Can you work these out from the model? Positions are in its coordinate system, mm. A direction names the side the tool comes from. Coordinates: 2 decimals unless noted, no trailing zeros. Order: outer loops, then holes, each group sorted by start corner. A loop starts at its lowest first (then second) coordinate and runs counter-clockwise, first axis right, second up. Notation, with made-up numbers: (-26, -19) -> (14, -19) arc R7 ccw to (14, -13) -> close; hole circle Ø1 at (85, 48). An arc over 180 degrees is marked (long way). Use a Markdown table: item, result. Add a question column.
1. If I drill on line 1 along Y through (x, z) = (-2.5, -4.25) (3 decimals); line 2 along X through (y, z) = (-20.5, -6); line 3 along Y through (x, z) = (-0.5, -4.25) (3 decimals), over which ranges is the centre line in solid material (lowest first)? Write a range as from..to.
2. For faces 1 (the cylindrical face through (-1.53, -22.37, -4.07)), 2 (the flat face through (-3, -14, -0.508)), 3 (the flat face through (-0.182, -21, -4)), 4 (the flat face through (-2, -25.175, -4)), 5 (the flat face through (-3.071, -19.626, 0.613)), which set-ups out of +Z, -Z, +X, -X, +Y, -Y let a thin tool reach every point of the face, with its end or its side?
3. For pin 1 Ø3 at (x, z) = (-2.5, -6) entering from -Y (3 decimals); pin 2 Ø3.5 at (x, y) = (-1.5, -6) entering from -Z; pin 3 Ø1.5 at (x, z) = (-1, -2.5) entering from +Y (3 decimals); pin 4 Ø3 at (x, y) = (-2, -20.5) entering from +Z, each with a flat end and sliding along its axis, tell me the tip position at first contact or that it passes through.
4. Suppose I cut it at C-C, the plane y = -21.35. List the corners of the cut face in (x, z) for me.
5. Suppose I cut it at B-B, the plane z = -3. List the corners of the cut face in (x, y) for me (3 decimals), then the cut area to 3 significant figures.
6. Suppose I cut it at A-A, the plane y = -10.75. List the corners of the cut face in (x, z) for me, then the cut area to 4 significant figures.
7. We'd pull the mould along X, two halves only. Please class faces 6 (the flat face through (-0.057, -21, 1)), 7 (the flat face through (-3.932, -21, -4)), 8 (the flat face through (-2, -25.85, 0)): pulls with the +X half, pulls with the -X half, needs draft (parallel to the pull), parting line crosses it, or undercut.
Autodesk Inventor part; units mm, degrees
ref_plane "YZ Plane" through (0, 0, 0) normal (1, 0, 0) x (0, 1, 0)
ref_plane "XZ Plane" through (0, 0, 0) normal (0, 1, 0) x (-1, 0, 0)
ref_plane "XY Plane" through (0, 0, 0) normal (0, 0, 1) x (1, 0, 0)
ref_plane "Work Plane3" through (0, -0.0002, 0) normal (0, 0, 1) x (1, 0, 0)
sketch "Sketch8" plane through (0, -0.0002, 0) normal (0, 0, 1) x (1, 0, 0)
  line L0 (-0.007, 0.0002) -> (-0.007, -15.3498)
  line L1 (-0.007, 0.0002) -> (-4.107, 0.0002)
  line L2 (-4.107, 0.0002) -> (-4.107, -11.3498)
  line L3 (-5.107, -11.3498) -> (0.993, -11.3498)
  line L4 (0.993, -11.3498) -> (0.993, 0.0002)
  line L5 (0.993, 0.0002) -> (-5.107, 0.0002)
  line L6 (-5.107, 0.0002) -> (-5.107, -11.3498)
  line L7 (-4.107, -11.3498) -> (-1.0868, -11.3498)
  point P0 (-4.107, 0.0002)
  point P1 (-0.007, 0.0002)
  point P2 (-0.007, -11.3498)
  dimension "d71" = 1
  dimension "d72" = 1
extrude "side" add sketch "Sketch8" along normal blind 1.5
sketch "Sketch14" plane through (0, -0.0002, 0) normal (0, 0, -1) x (-1, 0, 0)
  line L0 (-0.993, 0) -> (5.107, 0)
  line L1 (5.107, -11.3498) -> (-0.993, -11.3498)
  line L2 (5.107, 0.0002) -> (4.307, 0.0002)
  line L3 (4.307, 0.0002) -> (4.307, -11.3498)
  line L4 (4.307, -11.3498) -> (5.107, -11.3498)
  line L5 (5.107, -11.3498) -> (5.107, 0.0002)
  line L6 (-0.993, -11.3498) -> (-0.193, -11.3498)
  line L7 (-0.193, -11.3498) -> (-0.193, 0.0002)
  line L8 (-0.193, 0.0002) -> (-0.993, 0.0002)
  line L9 (-0.993, 0.0002) -> (-0.993, -11.3498)
  line L10 (4.107, 0.0002) -> (4.107, -11.3498)
  line L11 (0.007, 0.0002) -> (0.007, -15.3498)
  point P0 (0, 0.0002)
  point P1 (-0.993, 0.0002)
  point P2 (-0.993, 0.0002)
  point P3 (-0.193, 0.0002)
  point P4 (4.307, 0.0002)
  dimension "d73" = 0.2
  dimension "d74" = 0.2
extrude "side_tabs" add sketch "Sketch14" along normal blind 0.75 contours L0 L7 L1 L9 | L0 L5 L1 L3
sketch "Sketch15" plane through (-5.107, -11.35, 1.5) normal (0, -1, 0) x (1, 0, 0)
  line L0 (0.8, -1.5) -> (5.3, -1.5)
  line L1 (5.3, -1.5) -> (5.3, -2.25)
  line L2 (6.1, -2.25) -> (5.3, -2.25)
  line L3 (0, 0) -> (6.1, 0)
  line L4 (0.8, -2.25) -> (0, -2.25)
  line L5 (0.8, -1.5) -> (0.8, -2.25)
  line L6 (5.3, -1.5) -> (0.8, -1.5)
  line L7 (1, -1.5) -> (4.0182, -1.5)
  line L8 (0.8, -1.5) -> (0.8, -2.25)
  line L9 (0.8, -1.5) -> (3.8202, -1.5)
  line L10 (3.8202, -1.5) -> (3.8202, -2.008)
  line L11 (3.8202, -2.008) -> (0.8, -2.008)
  line L12 (0.8, -2.008) -> (0.8, -1.5)
  line L13 (6.1, -2.25) -> (6.1, 0)
  line L14 (0, 0) -> (0, -2.25)
  line L15 (4.0202, -1.5) -> (4.0202, -2.8009)
  point P0 (5.107, -1.5)
  point P1 (3.8202, -1.5)
  dimension "d99" = 0.508
  dimension "d100" = 0.2
extrude "fill_gaps" add sketch "Sketch15" along normal blind 14.5
sketch "Sketch16" plane through (-5.107, -25.85, 1.5) normal (0, -1, 0) x (1, 0, 0)
  line L0 (5.3, -2.25) -> (6.1, -2.25)
  line L1 (5.3, -1.5) -> (5.3, -2.25)
  line L2 (3.8202, -1.5) -> (5.3, -1.5)
  line L3 (3.8202, -2.008) -> (3.8202, -1.5)
  line L4 (0.8, -2.008) -> (3.8202, -2.008)
  line L5 (0.8, -2.25) -> (0.8, -2.008)
  line L6 (0, -2.25) -> (0.8, -2.25)
  line L7 (5.3, -2.25) -> (0.8, -2.25)
  point P0 (5.107, -1.5)
extrude "fill_gaps_2" add sketch "Sketch16" against normal blind 9.8
chamfer "Chamfer1" distance 2 angle 45 1 edges at (-2.057, 0, 1.5)
sketch "Sketch17" plane through (0, -0.0002, -0.75) normal (0, 0, -1) x (-1, 0, 0)
  line L0 (0.007, -17.3498) -> (0.007, -25.3498)
  line L1 (4.107, -17.3498) -> (0.007, -17.3498)
  line L2 (4.107, -25.3498) -> (4.107, -17.3498)
  line L3 (0.007, -25.3498) -> (4.107, -25.3498)
  line L4 (0.182, -25.1748) -> (3.932, -25.1748)
  line L5 (3.932, -25.1748) -> (3.932, -17.5248)
  line L6 (3.932, -17.5248) -> (0.182, -17.5248)
  line L7 (0.182, -17.5248) -> (0.182, -25.1748)
  point P0 (0, 0.0002)
  dimension "d86" = 0.175
  dimension "d87" = 0.175
  dimension "d88" = 0.175
  dimension "d89" = 0.175
extrude "sliding_block" add sketch "Sketch17" along normal blind 7.2 contours L7 L6 L5 L4
ref_plane "Work Plane4" through (-2.2725, -22.3901, 1.5) normal (0, 0, 1) x (1, 0, 0)
sketch "Sketch19" plane through (-2.2725, -22.3901, 1.5) normal (0, 0, 1) x (1, 0, 0)
  circle A0 centre (0.2155, 1.0401) radius 1.15
  point P0 (2.2725, 22.3901)
extrude "screw_hole" cut sketch "Sketch19" against normal through all
sketch "Sketch20" plane through (0, -0.0002, 1.5) normal (0, 0, 1) x (1, 0, 0)
  line L0 (-2.057, -19.0404) -> (-0.057, -20.1951)
  line L1 (-0.057, -20.1951) -> (-0.057, -22.5045)
  line L2 (-0.057, -22.5045) -> (-2.057, -23.6592)
  line L3 (-2.057, -23.6592) -> (-4.057, -22.5045)
  line L4 (-4.057, -22.5045) -> (-4.057, -20.1951)
  line L5 (-4.057, -20.1951) -> (-2.057, -19.0404)
  circle A0 centre (-2.057, -21.3498) radius 1.15
  point P0 (0, 0.0002)
  dimension "d102" = 4
extrude "nut_slot" cut sketch "Sketch20" against normal blind 1.8 contours L0 L1 L2 L3 L4 L5 | A0
equation "\"d73\" = d74"
equation "\"d86\" = d89"
equation "\"d87\" = d89"
equation "\"d88\" = d89"
properties part number "surgical_holder_side2"
Worked out:
| question | item | result |
|---|---|---|
| 1 | line 1 | y = -25.175..-22.411, -20.289..-17.525 |
| 1 | line 2 | x = -3.93..-2.83, -1.28..-0.18 |
| 1 | line 3 | y = -25.175..-17.525 |
| 2 | face 1 | +Z, -Z |
| 2 | face 2 | -Z, +Y |
| 2 | face 3 | -Z, +X, +Y, -Y |
| 2 | face 4 | -Z, +X, -X, -Y |
| 2 | face 5 | +Z |
| 3 | pin 1 | stops at y = -25.175 |
| 3 | pin 2 | stops at z = -0.75 |
| 3 | pin 3 | stops at y = -17.525 |
| 3 | pin 4 | stops at z = 1.5 |
| 4 | outline | (-5.11, -0.75) -> (-3.93, -0.75) -> (-3.93, -7.95) -> (-3.21, -7.95) -> (-3.21, -0.3) -> (-4.06, -0.3) -> (-4.06, 1.5) -> (-5.11, 1.5) -> close; (-0.91, -7.95) -> (-0.18, -7.95) -> (-0.18, -0.75) -> (0.99, -0.75) -> (0.99, 1.5) -> (-0.06, 1.5) -> (-0.06, -0.3) -> (-0.91, -0.3) -> close |
| 5 | outline | (-3.932, -25.175) -> (-0.182, -25.175) -> (-0.182, -17.525) -> (-3.932, -17.525) -> close; hole circle Ø2.3 at (-2.057, -21.35) |
| 5 | area | 24.5 mm² |
| 6 | outline | (-5.11, -0.75) -> (-4.31, -0.75) -> (-4.31, 0) -> (0.19, 0) -> (0.19, -0.75) -> (0.99, -0.75) -> (0.99, 1.5) -> (-5.11, 1.5) -> close |
| 6 | area | 10.35 mm² |
| 7 | face 6 | undercut |
| 7 | face 7 | pulls with the -X half |
| 7 | face 8 | needs draft |
